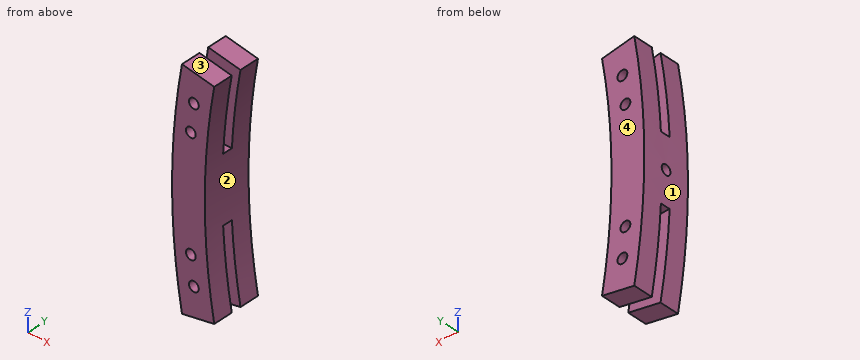
```python
from build123d import *

# Parameters (mm, degrees)
BASE_DEPTH            = 7.5
MOUNT_START           = -1.5
MOUNT_DEPTH           = 3
MOUNT_HOLE_DEPTH      = 204.131478566
MOUNT_HOLE_DEPTH_BACK = 204.131478566
SKETCH12_R            = 1.5
SKETCH14_R            = 1.5
SHAFT_HOLE_DEPTH      = 37.394984425
SKETCH13_W            = 2.5
SKETCH13_H            = 3


with BuildPart() as part:
    # Sketch9 → base (new, symmetric)
    with BuildSketch(Plane(origin=(0, 0, 0), x_dir=(1, 0, 0), z_dir=(0, 1, 0))):
        with BuildLine():
            ThreePointArc((-187.113473072, -32.993153757), (-190, 0), (-187.113473072, 32.993153757))
            Line((-187.113473072, 32.993153757), (-196.961550602, 34.729635533))
            ThreePointArc((-196.961550602, 34.729635533), (-200, 0), (-196.961550602, -34.729635533))
            Line((-196.961550602, -34.729635533), (-187.113473072, -32.993153757))
        make_face()
    extrude(amount=BASE_DEPTH, both=True)

    # Sketch11 → mount (cut)
    with BuildSketch(Plane(origin=(0, 0, 0), x_dir=(1, 0, 0), z_dir=(0, 1, 0)).offset(MOUNT_START)):
        with BuildLine():
            Line((-189.73665961, -10), (-199.749843554, -10))
            ThreePointArc((-199.749843554, -10), (-198.7407137, -22.408228804), (-196.961550602, -34.729635533))
            Line((-196.961550602, -34.729635533), (-187.113473072, -32.993153757))
            ThreePointArc((-187.113473072, -32.993153757), (-188.775466906, -21.536552519), (-189.73665961, -10))
        make_face()
        with BuildLine():
            Line((-189.73665961, 10), (-199.749843554, 10))
            ThreePointArc((-199.749843554, 10), (-198.7407137, 22.408228804), (-196.961550602, 34.729635533))
            Line((-196.961550602, 34.729635533), (-187.113473072, 32.993153757))
            ThreePointArc((-187.113473072, 32.993153757), (-188.775466906, 21.536552519), (-189.73665961, 10))
        make_face()
    extrude(amount=MOUNT_DEPTH, mode=Mode.SUBTRACT)

    # Sketch12 → mount hole (cut, two sides: drawn at the far end of the back side and taken through both)
    with BuildSketch(Plane(origin=(0, 0, 0), x_dir=(1, 0, 0), z_dir=(0, 1, 0)).offset(-MOUNT_HOLE_DEPTH_BACK)):
        with Locations(Location((-193.331747968, 25.452607483, 0), (0, 0, 270))):
            Circle(SKETCH12_R)
        with Locations(Location((-194.257966128, 16.995369836, 0), (0, 0, 270))):
            Circle(SKETCH12_R)
        with Locations(Location((-194.257966128, -16.995369836, 0), (0, 0, 270))):
            Circle(SKETCH12_R)
        with Locations(Location((-193.331747968, -25.452607483, 0), (0, 0, 270))):
            Circle(SKETCH12_R)
    extrude(amount=MOUNT_HOLE_DEPTH + MOUNT_HOLE_DEPTH_BACK, mode=Mode.SUBTRACT)

    # Sketch14 → shaft hole (cut, through all)
    with BuildSketch(Plane.ZY.offset(195)):
        with Locations(Location((0, 0, 0), (0, 0, 90))):
            Circle(SKETCH14_R)
    extrude(amount=SHAFT_HOLE_DEPTH, mode=Mode.SUBTRACT)

    # Sketch13 → bearing hole (revolve, cut)
    with BuildSketch(Plane(origin=(0, 0, 0), x_dir=(1, 0, 0), z_dir=(0, 1, 0)), mode=Mode.PRIVATE) as bearing_hole_sk:
        with Locations((-195, 1.5)):
            Rectangle(SKETCH13_W, SKETCH13_H)
    revolve(bearing_hole_sk.sketch.rotate(Axis((0, 0, 0), (-1, 0, 0)), 270), axis=Axis((0, 0, 0), (-1, 0, 0)), mode=Mode.SUBTRACT)


solid = part.part
```
Geometry: final body of the model. Coordinates: model frame, mm. Face numbers are marked on the shaded views. Round coordinates to 2 decimals unless told otherwise and drop trailing zeros. Loops run counter-clockwise (first coordinate to the right, second up) from the corner with the lowest first, then second, coordinate; pieces in that order, holes last. Notation, with made-up numbers: (11.25, 86) -> (53.25, 86) arc R14 cw to (53.25, 111) -> close; hole circle Ø4 at (22, -2.75). An arc over 180 degrees is marked (long way). Use one line per item in the form item = value. Start each with the question number.
1) Line query: L1, parallel to Z at x = -194.85, y = 0; L2, parallel to Y at x = -196.25, z = -18.5; L3, parallel to Z at x = -198.2, y = 0. Output: solid intervals per line, ascending.
2) Section B-B on x = -188.25. Output: boundary loops of the cut face in (y, z).
3) Section A-A on z = 0. Output: boundary loops of the cut face in (x, y), then the cut area to 3 significant figures.
4) Draft query along Z for the marked faces 1, 2, 3 and 4. Return one class per face: released by +Z, released by -Z, zero draft, split by the parting line, or undercut.
5) First-contact query: P1, Ø1.5, axis at x = -193.5, y = 0.5, coming from the +Z side; P2, Ø1, axis at y = 1.5, z = 1.5, coming from the +X side; P3, Ø2.5, axis at y = 0, z = 0, coming from the -X side. Flat tips, straight axial feed; report the tip coordinate or a pass-through.
6) Section C-C on x = -191. Output: boundary loops of the cut face in (y, z), then the cut area to 3 significant figures.
Response:
q1.L1 = -10 to -3, 3 to 10
q1.L2 = -7.5 to -1.5, 1.5 to 7.5
q1.L3 = -10 to -1.5, 1.5 to 10
q2.outline = (-7.5, -33.19) -> (-1.5, -33.19) -> (-1.5, -25.73) -> (-7.5, -25.73) -> close; (-7.5, 25.73) -> (-1.5, 25.73) -> (-1.5, 33.19) -> (-7.5, 33.19) -> close; (1.5, -33.19) -> (7.5, -33.19) -> (7.5, -25.73) -> (1.5, -25.73) -> close; (1.5, 25.73) -> (7.5, 25.73) -> (7.5, 33.19) -> (1.5, 33.19) -> close
q3.outline = (-200, -7.5) -> (-190, -7.5) -> (-190, 7.5) -> (-200, 7.5) -> (-200, 1.5) -> (-196.25, 1.5) -> (-196.25, 3) -> (-193.75, 3) -> (-193.75, -3) -> (-196.25, -3) -> (-196.25, -1.5) -> (-200, -1.5) -> close
q3.area = 124 mm^2
q4.face_1 = split by the parting line
q4.face_2 = undercut
q4.face_3 = released by +Z
q4.face_4 = zero draft
q5.P1 = 10
q5.P2 = -189.99
q5.P3 = -193.75
q6.outline = (-7.5, -33.68) -> (-1.5, -33.68) -> (-1.5, -10) -> (1.5, -10) -> (1.5, -33.68) -> (7.5, -33.68) -> (7.5, 33.68) -> (1.5, 33.68) -> (1.5, 10) -> (-1.5, 10) -> (-1.5, 33.68) -> (-7.5, 33.68) -> close
q6.area = 868 mm^2
